Geometry check sheet. Reference: the model listing, model coordinates, mm. Coordinates: 2 decimals unless noted, no trailing zeros. Order: outer loops, then holes, each group sorted by start corner. A loop starts at its lowest first (then second) coordinate and runs counter-clockwise, first axis right, second up. Notation, with made-up numbers: (-24.5, 65) - (-16.5, 65) arc R21 ccw to (-16.5, 82) - close; hole circle Ø9 at (50.25, 70.25). An arc over 180 degrees is marked (long way). Put each result on its own line as item: value.
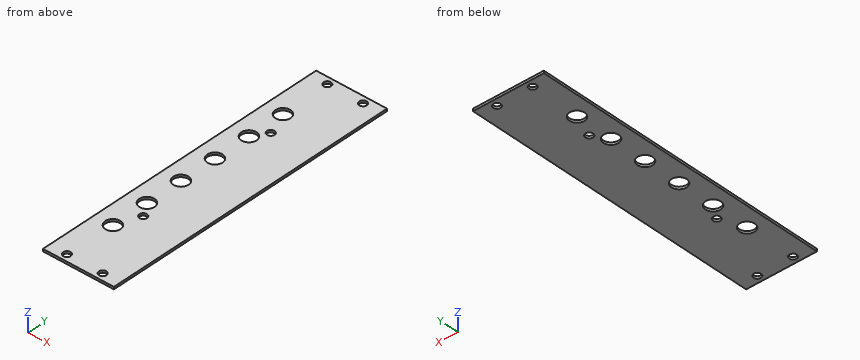
from build123d import *

# Parameters (mm, degrees)
SKETCH2_W                        = 30.24
SKETCH2_H                        = 128.5
SKETCH2_R                        = 1.6
BOSS_EXTRUDE1_DEPTH              = 1
SMA_CUTS_DEPTH                   = 133.014043192
SMA_CUTS_DEPTH_BACK              = 133.014043192
SKETCH3_R                        = 3.25
MOUNTING_BRACKET_CUTS_DEPTH      = 133.014043192
MOUNTING_BRACKET_CUTS_DEPTH_BACK = 133.014043192
SKETCH4_R                        = 1.6


with BuildPart() as part:
    # Sketch2 → Boss-Extrude1 (new body)
    with BuildSketch(Plane.XY):
        with Locations((15.12, 64.25)):
            Rectangle(SKETCH2_W, SKETCH2_H)
        with Locations((7.5, 3)):
            Circle(SKETCH2_R, mode=Mode.SUBTRACT)
        with Locations((22.74, 3)):
            Circle(SKETCH2_R, mode=Mode.SUBTRACT)
        with Locations((22.74, 125.5)):
            Circle(SKETCH2_R, mode=Mode.SUBTRACT)
        with Locations((7.5, 125.5)):
            Circle(SKETCH2_R, mode=Mode.SUBTRACT)
    extrude(amount=BOSS_EXTRUDE1_DEPTH)

    # Sketch3 → sma_cuts (cut, two sides: drawn at the far end of the back side and taken through both)
    with BuildSketch(Plane.XY.offset(1).offset(-SMA_CUTS_DEPTH_BACK)):
        with Locations((7.85, 104.25)):
            Circle(SKETCH3_R)
        with Locations((7.85, 88.25)):
            Circle(SKETCH3_R)
        with Locations((7.85, 72.25)):
            Circle(SKETCH3_R)
        with Locations((7.85, 56.25)):
            Circle(SKETCH3_R)
        with Locations((7.85, 40.25)):
            Circle(SKETCH3_R)
        with Locations((7.85, 24.25)):
            Circle(SKETCH3_R)
    extrude(amount=SMA_CUTS_DEPTH + SMA_CUTS_DEPTH_BACK, mode=Mode.SUBTRACT)

    # Sketch4 → mounting_bracket_cuts (cut, two sides: drawn at the far end of the back side and taken through both)
    with BuildSketch(Plane.XY.offset(1).offset(-MOUNTING_BRACKET_CUTS_DEPTH_BACK)):
        with Locations((11.7314, 94.225)):
            Circle(SKETCH4_R)
        with Locations((11.7314, 34.225)):
            Circle(SKETCH4_R)
    extrude(amount=MOUNTING_BRACKET_CUTS_DEPTH + MOUNTING_BRACKET_CUTS_DEPTH_BACK, mode=Mode.SUBTRACT)


solid = part.part
Q1. Thickness scan on L1, parallel to X at y = 125.5, z = 0.4; L2, parallel to X at y = 56.25, z = 0.35; L3, parallel to Y at x = 11.5, z = 0.8. Record the ranges inside material, lowest first. Write a range as [from, to].
Answer block:
L1: x = [0, 5.9], [9.1, 21.14], [24.34, 30.24]
L2: x = [0, 4.6], [11.1, 30.24]
L3: y = [0, 32.64], [35.81, 92.64], [95.81, 128.5]
Q2. Section check C-C on x = 7.5. State how many separate pieces and enclosed holes the cut face has, then the cut area to 3 significant figures.
Answer block:
separate pieces: 9
enclosed holes: 0
area: 83.3 mm^2
Q3. Section check A-A on y = 72.25. Record the boundary of the cut face in (x, z).
Answer block:
outline: (0, 0) - (4.6, 0) - (4.6, 1) - (0, 1) - close; (11.1, 0) - (30.24, 0) - (30.24, 1) - (11.1, 1) - close
Q4. Section check B-B on y = 3. Record the boundary of the cut face in (x, z), then the cut area to 3 significant figures.
Answer block:
outline: (0, 0) - (5.9, 0) - (5.9, 1) - (0, 1) - close; (9.1, 0) - (21.14, 0) - (21.14, 1) - (9.1, 1) - close; (24.34, 0) - (30.24, 0) - (30.24, 1) - (24.34, 1) - close
area: 23.8 mm^2
